from build123d import *

# Parameters (mm, degrees)
SKETCH_1_W          = 150
SKETCH_1_H          = 95.25
EXTRUDE_1_DEPTH     = 3
SKETCH_1_3_W        = 21.6
SKETCH_1_3_H        = 27.1
CUT_EXTRUDE_2_DEPTH = 3


with BuildPart() as part:
    # Sketch 1 → Extrude 1 (new body)
    with BuildSketch(Plane.XY):
        Rectangle(SKETCH_1_W, SKETCH_1_H)
    extrude(amount=EXTRUDE_1_DEPTH)

    # Sketch 1_3 → Cut-Extrude 2 (cut)
    with BuildSketch(Plane.XY):
        with Locations((-37.4, 0)):
            Rectangle(SKETCH_1_3_W, SKETCH_1_3_H)
        with BuildLine():
            Line((3.2, 14.5), (45.2, 14.5))
            ThreePointArc((45.2, 14.5), (47.321320344, 13.621320344), (48.2, 11.5))
            Line((48.2, 11.5), (48.2, -11.5))
            ThreePointArc((48.2, -11.5), (47.321320344, -13.621320344), (45.2, -14.5))
            Line((45.2, -14.5), (3.2, -14.5))
            ThreePointArc((3.2, -14.5), (1.078679656, -13.621320344), (0.2, -11.5))
            Line((0.2, -11.5), (0.2, 11.5))
            ThreePointArc((0.2, 11.5), (1.078679656, 13.621320344), (3.2, 14.5))
        make_face()
    extrude(amount=CUT_EXTRUDE_2_DEPTH, mode=Mode.SUBTRACT)


solid = part.part
Here's how the part is built. I have some questions about the finished solid (model axes, mm). A direction names the side the tool comes from. Give positions to 0.01 mm unless a question says otherwise; leave off trailing zeros. Order: outer loops, then holes, each group sorted by start corner. A loop starts at its lowest first (then second) coordinate and runs counter-clockwise, first axis right, second up. Notation, with made-up numbers: M -37,5.5 L 16,5.5 A15 cw 16,23.5 Z; hole C 59.5,35 d7. An arc over 180 degrees is marked long. Answer as a JSON object with one key per item and string values. Group by question number.
1) Suppose I cut it at B-B, the plane y = 1. Write out the boundary of the cut face in (x, z).
2) Suppose I cut it at A-A, the plane x = -39. Write out the boundary of the cut face in (y, z) (3 decimals).
3) We'd pull the mould along X, two halves only. Please class faces 3 (the flat face through (-75, -1, 1)), 4 (the flat face through (75, -1, 1)), 5 (the flat face through (0.2, 0, 1)): pulls with the +X half, pulls with the -X half, needs draft (parallel to the pull), parting line crosses it, or undercut.
4) Suppose I cut it at C-C, the plane z = 2.25. Write out the boundary of the cut face in (x, y) (3 decimals), plus the area to 3 significant figures.
5) Please list where these lines run through material, in increasing order: L1, parallel to X at y = -5, z = 2.7; L2, parallel to X at y = -13.5, z = 1.4; L3, parallel to Y at x = -43.5, z = 2.1 (3 decimals). Write a range as [from, to].
6) On a 3-axis mill with a long thin cutter (end or side, diameter ignored), from which of +Z, -Z, +X, -X, +Y, -Y can I reach the whole of each face in a straight line? I mean faces 1 (the flat face through (-38, 13.55, 1)), 2 (the flat face through (-1, 47.625, 1)). Say none if no direction works.
Results found:
{
 "1": {"outline": "M -75,0 L -48.2,0 L -48.2,3 L -75,3 Z; M -26.6,0 L 0.2,0 L 0.2,3 L -26.6,3 Z; M 48.2,0 L 75,0 L 75,3 L 48.2,3 Z"},
 "2": {"outline": "M -47.625,0 L -13.55,0 L -13.55,3 L -47.625,3 Z; M 13.55,0 L 47.625,0 L 47.625,3 L 13.55,3 Z"},
 "3": {"face 3": "pulls with the -X half", "face 4": "pulls with the +X half", "face 5": "undercut"},
 "4": {"outline": "M -75,-47.625 L 75,-47.625 L 75,47.625 L -75,47.625 Z; hole M -48.2,-13.55 L -26.6,-13.55 L -26.6,13.55 L -48.2,13.55 Z; hole M 0.2,-11.5 A3 ccw 3.2,-14.5 L 45.2,-14.5 A3 ccw 48.2,-11.5 L 48.2,11.5 A3 ccw 45.2,14.5 L 3.2,14.5 A3 ccw 0.2,11.5 Z", "area": "12,300 mm²"},
 "5": {"L1": "[-75, -48.2], [-26.6, 0.2], [48.2, 75]", "L2": "[-75, -48.2], [-26.6, 0.96], [47.44, 75]", "L3": "[-47.625, -13.55], [13.55, 47.625]"},
 "6": {"face 1": "+Z, -Z", "face 2": "+Z, -Z, +X, -X, +Y"}
}
